Model file for the job. Use its own axes, mm. Give positions to 0.01 mm unless a question says otherwise; leave off trailing zeros. Loops run counter-clockwise (first coordinate to the right, second up) from the corner with the lowest first, then second, coordinate; pieces in that order, holes last. Notation, with made-up numbers: (30, -38.75) - (70, -38.75) arc R29 ccw to (70, -4.75) - close; hole circle Ø8 at (33.25, 6). An arc over 180 degrees is marked (long way). Answer as CSV lines item,"result". Start each with the question number.
Item 1: Saw through at A-A on y = -6.15. Give the cut face in (x, z).
Item 2: Pin check, flat tip, straight feed: pin 1 (1 mm diameter, centred on y = -28, z = 0.5, fed in from -X). Stop position of the tip, or through.
Item 3: Drill centre lines: L1, parallel to Y at x = 5, z = 0.95; L2, parallel to X at y = -40.5, z = 1.5; L3, parallel to X at y = -6.5, z = 0.9. Where is each one in solid material? Low to high. Write a range as from..to.
Item 4: Saw through at D-D on y = -30.5. Give the cut face in (x, z).
Item 5: Saw through at B-B on y = -40.5. Give the cut face in (x, z), plus the area to 3 significant figures.
Item 6: Saw through at C-C on y = 9.85. Give the cut face in (x, z).
from build123d import *

# Parameters (mm, degrees)
BOSS_EXTRU_1_DEPTH      = 2
ESQUISSE2_R             = 0.9
ENL_V_MAT_EXTRU_1_DEPTH = 51.356664533
ESQUISSE3_R             = 0.9
ENL_V_MAT_EXTRU_2_DEPTH = 51.356664533


with BuildPart() as part:
    # Esquisse1 → Boss.-Extru.1 (new body)
    with BuildSketch(Plane.XY):
        with BuildLine():
            Line((-22.3, -14.668472775), (-22.3, -44))
            Line((-22.3, -44), (4, -44))
            Line((4, -44), (4, -21.327759335))
            ThreePointArc((4, -21.327759335), (-1.668200766, 11.550292485), (-22.3, -14.668472775))
        make_face()
    extrude(amount=BOSS_EXTRU_1_DEPTH)

    # Esquisse2 → Enlèv. mat.-Extru.1 (cut, through all)
    with BuildSketch(Plane.XY.offset(2)):
        with Locations((9.85, -6.15)):
            Circle(ESQUISSE2_R)
        with Locations((5.163708499, -17.463708499)):
            Circle(ESQUISSE2_R)
        with Locations((-22.15, -6.15)):
            Circle(ESQUISSE2_R)
        with Locations((-17.463708499, 5.163708499)):
            Circle(ESQUISSE2_R)
        with Locations((-6.15, 9.85)):
            Circle(ESQUISSE2_R)
        with Locations((5.163708499, 5.163708499)):
            Circle(ESQUISSE2_R)
    extrude(amount=-ENL_V_MAT_EXTRU_1_DEPTH, mode=Mode.SUBTRACT)

    # Esquisse3 → Enlèv. mat.-Extru.2 (cut, through all)
    with BuildSketch(Plane(origin=(0, 0, 0), x_dir=(-1, 0, 0), z_dir=(0, 0, -1))):
        with Locations((5.77, -40.5)):
            Circle(ESQUISSE3_R)
    extrude(amount=-ENL_V_MAT_EXTRU_2_DEPTH, mode=Mode.SUBTRACT)


solid = part.part
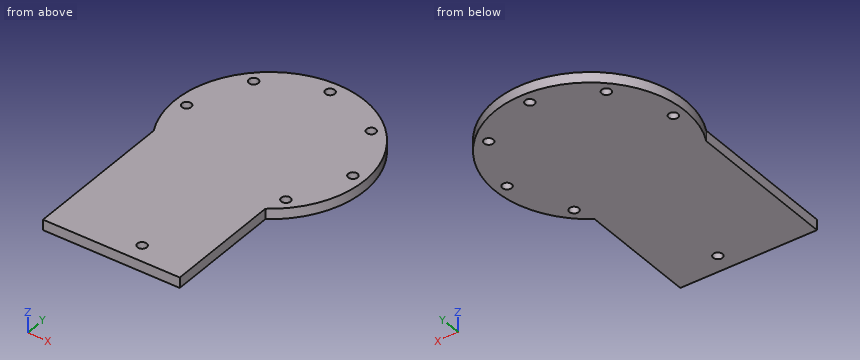
Responses:
1,outline,"(-24.41, 0) - (-23.05, 0) - (-23.05, 2) - (-24.41, 2) - close; (-21.25, 0) - (8.95, 0) - (8.95, 2) - (-21.25, 2) - close; (10.75, 0) - (12.11, 0) - (12.11, 2) - (10.75, 2) - close"
2,pin 1,"x = -22.3"
3,L1,"-20.61..-18.35, -16.58..4.28, 6.05..8.31"
3,L2,"-22.3..-6.67, -4.87..4"
3,L3,"-24.41..-22.98, -21.32..9.02, 10.68..12.11"
4,outline,"(-22.3, 0) - (4, 0) - (4, 2) - (-22.3, 2) - close"
5,outline,"(-22.3, 0) - (-6.67, 0) - (-6.67, 2) - (-22.3, 2) - close; (-4.87, 0) - (4, 0) - (4, 2) - (-4.87, 2) - close"
5,area,"49.0 mm2"
6,outline,"(-14.95, 0) - (-7.05, 0) - (-7.05, 2) - (-14.95, 2) - close; (-5.25, 0) - (2.65, 0) - (2.65, 2) - (-5.25, 2) - close"
